from build123d import *

# Parameters (mm, degrees)
BOSS_EXTRUDE1_DEPTH             = 2.38125
SKETCH2_R                       = 38.608
SKETCH2_R_2                     = 8.73125
CUT_EXTRUDE1_DEPTH              = 2.38125
SKETCHED_START                  = 31.75
SKETCHED_BEND1_DEPTH            = 50.8
SKETCHED_BEND1_2_DEPTH          = 50.8
SKETCHED_BEND2_DEPTH            = 50.8
SKETCHED_BEND2_2_DEPTH          = 50.8
TAP_DRILL_FOR_M3X0_5_TAP1_D     = 2.5
TAP_DRILL_FOR_M3X0_5_TAP1_DEPTH = 2.38125
TAP_DRILL_FOR_M3X0_5_TAP2_D     = 2.5


# Read off the part's stored shape, not the designer's step: Sketched Bend1, Sketched Bend2
with BuildPart() as part:
    # Sketch1 → Boss-Extrude1 (new body)
    with BuildSketch(Plane.XY):
        Polygon((-55.274119317, 31.75), (-10.824119317, 31.75), (29.9865, 9.525), (68.0865, 9.525), (108.897119317, 31.75), (153.347119317, 31.75), (153.347119317, 82.55), (108.897119317, 82.55), (68.0865, 104.775), (29.9865, 104.775), (-10.824119317, 82.55), (-55.274119317, 82.55), align=None)
    extrude(amount=BOSS_EXTRUDE1_DEPTH)

    # Sketch2 → Cut-Extrude1 (cut)
    with BuildSketch(Plane(origin=(0, 0, 0), x_dir=(-1, 0, 0), z_dir=(0, 0, -1))):
        with Locations((-49.1, 57.15)):
            Circle(SKETCH2_R)
        with Locations((-117.15, 57.15)):
            Circle(SKETCH2_R_2)
        with Locations((18.95, 57.15)):
            Circle(SKETCH2_R_2)
    extrude(amount=-CUT_EXTRUDE1_DEPTH, mode=Mode.SUBTRACT)

    # Sketched Bend1 outline → Sketched Bend1 (cut)
    with BuildSketch(Plane(origin=(0, 0, 0), x_dir=(1, 0, 0), z_dir=(0, 1, 0)).offset(SKETCHED_START)):
        with BuildLine():
            Line((153.347119317, 0), (142.825615918, 0))
            ThreePointArc((142.825615918, 0), (140.837913282, -1.750089228), (138.265869317, -2.38125))
            Line((138.265869317, -2.38125), (153.347119317, -2.38125))
            Line((153.347119317, -2.38125), (153.347119317, 0))
        make_face()
    extrude(amount=SKETCHED_BEND1_DEPTH, mode=Mode.SUBTRACT)

    # Sketched Bend1 2 outline → Sketched Bend1 2 (add)
    with BuildSketch(Plane(origin=(0, 0, 0), x_dir=(1, 0, 0), z_dir=(0, 1, 0)).offset(SKETCHED_START)):
        with BuildLine():
            Line((143.822119317, 3.175), (143.822119317, 11.398742286))
            Line((143.822119317, 11.398742286), (141.440869317, 11.398742286))
            Line((141.440869317, 11.398742286), (141.440869317, 3.175))
            ThreePointArc((141.440869317, 3.175), (140.510933348, 0.929935969), (138.265869317, 0))
            Line((138.265869317, 0), (142.825615918, 0))
            ThreePointArc((142.825615918, 0), (143.567143037, 1.511145738), (143.822119317, 3.175))
        make_face()
    extrude(amount=SKETCHED_BEND1_2_DEPTH)

    # Sketched Bend2 outline → Sketched Bend2 (cut)
    with BuildSketch(Plane(origin=(0, 0, 0), x_dir=(1, 0, 0), z_dir=(0, 1, 0)).offset(SKETCHED_START)):
        with BuildLine():
            ThreePointArc((-40.065869317, -2.38125), (-42.637913282, -1.750089228), (-44.625615918, 0))
            Line((-44.625615918, 0), (-55.274119317, 0))
            Line((-55.274119317, 0), (-55.274119317, -2.38125))
            Line((-55.274119317, -2.38125), (-40.065869317, -2.38125))
        make_face()
    extrude(amount=SKETCHED_BEND2_DEPTH, mode=Mode.SUBTRACT)

    # Sketched Bend2 2 outline → Sketched Bend2 2 (add)
    with BuildSketch(Plane(origin=(0, 0, 0), x_dir=(1, 0, 0), z_dir=(0, 1, 0)).offset(SKETCHED_START)):
        with BuildLine():
            ThreePointArc((-40.065869317, 0), (-42.310933347, 0.92993597), (-43.240869317, 3.175))
            Line((-43.240869317, 3.175), (-43.240869317, 11.525742286))
            Line((-43.240869317, 11.525742286), (-45.622119317, 11.525742286))
            Line((-45.622119317, 11.525742286), (-45.622119317, 3.175))
            ThreePointArc((-45.622119317, 3.175), (-45.367143037, 1.511145738), (-44.625615918, 0))
            Line((-44.625615918, 0), (-40.065869317, 0))
        make_face()
    extrude(amount=SKETCHED_BEND2_2_DEPTH)

    # Tap Drill for M3x0.5 Tap1
    with Locations(Plane(origin=(143.822119317, 0, 0), x_dir=(0, 0, -1), z_dir=(1, 0, 0))):
        with Locations((6.35, 76.2), (6.35, 38.1)):
            Hole(TAP_DRILL_FOR_M3X0_5_TAP1_D / 2, depth=TAP_DRILL_FOR_M3X0_5_TAP1_DEPTH)

    # Tap Drill for M3x0.5 Tap2 (through all)
    with Locations(Plane.ZY.offset(45.622119317)):
        with Locations((-6.35, 76.2), (-6.35, 38.1)):
            Hole(TAP_DRILL_FOR_M3X0_5_TAP2_D / 2)


solid = part.part
Can you work these out from the model? Positions are in its coordinate system, mm. A direction names the side the tool comes from. Coordinates: 2 decimals unless noted, no trailing zeros. Order: outer loops, then holes, each group sorted by start corner. A loop starts at its lowest first (then second) coordinate and runs counter-clockwise, first axis right, second up. Notation, with made-up numbers: M 2,74.25 L 45,74.25 A17 cw 45,102.25 Z; hole C 66.25,25 d3. An arc over 180 degrees is marked long. Write item = value, one per line.
(1) Suppose I cut it at D-D on x = -31. Please give me the cut outline in (y, z).
Results are:
outline = M 31.75,0 L 82.55,0 L 82.55,2.38 L 31.75,2.38 Z
(2) I need wall thicknesses on line 1 along Y through (x, z) = (143, -6.35); line 2 along X through (y, z) = (69.5, -4); line 3 along Y through (x, z) = (-18.95, 1.1). Which ranges of each line are inside material? Lowest first, please. Write a range as [from, to].
Results are:
line_1 = [31.75, 36.85], [39.35, 74.95], [77.45, 82.55]
line_2 = [-45.62, -43.24], [141.44, 143.82]
line_3 = [31.75, 48.42], [65.88, 82.55]
(3) For faces 4 (the face through (-32, 82.55, 1)), 5 (the face through (-43.241, 57, -7)), 6 (the face through (129, 31.75, 1)), 7 (the face through (129, 82.55, 1)), 8 (the face through (-32, 31.75, 1)), which set-ups out of +Z, -Z, +X, -X, +Y, -Y let a thin tool reach every point of the face, with its end or its side?
Results are:
face_4 = +Z, -Z, -X, +Y
face_5 = -Z, +Y, -Y
face_6 = +Z, -Z, +X, -Y
face_7 = +Z, -Z, +X, +Y
face_8 = +Z, -Z, -X, -Y
(4) For pin 1 Ø20 at (x, y) = (-18.95, 57.15) entering from -Z; pin 2 Ø1.2 at (x, y) = (142.5, 65) entering from -Z; pin 3 Ø2 at (y, z) = (67, -0.5) entering from -X, each with a flat end and sliding along its axis, tell me the tip position at first contact or that it passes through.
Results are:
pin_1 = 0
pin_2 = -11.4
pin_3 = -45.36
(5) Suppose I cut it at A-A on y = 57.15. State how many separate pieces and enclosed holes the cut face has, plus the area to 3 significant figures.
Results are:
separate_pieces = 4
enclosed_holes = 0
area = 230 mm2
(6) If we mould it in two halves opening along X, with no side actions, what happens to faces 1 (the face through (-45.622, 57, -7)), 2 (the face through (88.206, 20.482, 1.174)), 3 (the face through (141.441, 57, -7))? For each: pulls with the +X half, pulls with the -X half, needs draft (parallel to the pull), parting line crosses it, or undercut.
Results are:
face_1 = pulls with the -X half
face_2 = pulls with the +X half
face_3 = undercut
(7) Suppose I cut it at B-B on x = 49.1. Please give me the cut outline in (y, z) (3 decimals), plus the area to 3 significant figures.
Results are:
outline = M 9.525,0 L 18.542,0 L 18.542,2.381 L 9.525,2.381 Z; M 95.758,0 L 104.775,0 L 104.775,2.381 L 95.758,2.381 Z
area = 42.9 mm2
(8) Suppose I cut it at C-C on y = 29. Please give me the cut outline in (x, z), plus the area to 3 significant figures.
Results are:
outline = M -5.77,0 L 22.68,0 L 22.68,2.38 L -5.77,2.38 Z; M 75.52,0 L 103.85,0 L 103.85,2.38 L 75.52,2.38 Z
area = 135 mm2
